```python
from build123d import *

# Parameters (mm, degrees)
P_IDAT_VYSUNUT_M1_DEPTH  = 22
ZAOBLIT1_R               = 3
SKICA2_W                 = 107.918638888
SKICA2_H                 = 41.380791124
P_IDAT_VYSUNUT_M2_DEPTH  = 2
SKICA3_R                 = 2.425
ODEBRAT_VYSUNUT_M1_DEPTH = 8.5


with BuildPart() as part:
    # Skica1 → Přidat vysunutím1 (new body)
    with BuildSketch(Plane.XY):
        Polygon((0, 0), (101.3, 0), (99.05, 33.2), (2.25, 33.2), align=None)
    extrude(amount=P_IDAT_VYSUNUT_M1_DEPTH)

    # Zaoblit1
    zaoblit1_edges = [part.edges().sort_by_distance(p)[0] for p in [
        (2.25, 33.2, 11),
        (99.05, 33.2, 11),
    ]]
    fillet(zaoblit1_edges, radius=ZAOBLIT1_R)

    # Skica2 → Přidat vysunutím2 (add)
    with BuildSketch(Plane(origin=(0, 0, 0), x_dir=(-1, 0, 0), z_dir=(0, 0, -1))):
        with Locations((-50.804022796, 17.445366235)):
            Rectangle(SKICA2_W, SKICA2_H)
    extrude(amount=P_IDAT_VYSUNUT_M2_DEPTH)

    # Skica3 → Odebrat vysunutím1 (cut)
    with BuildSketch(Plane.XY.offset(22)):
        with Locations((57.79, 9.455)):
            Circle(SKICA3_R)
        with Locations(Location((43.51, 9.455, 0), (0, 0, 180))):
            Circle(SKICA3_R)
        with Locations(Location((57.79, 23.735, 0), (0, 0, 180))):
            Circle(SKICA3_R)
        with Locations((43.51, 23.735)):
            Circle(SKICA3_R)
    extrude(amount=-ODEBRAT_VYSUNUT_M1_DEPTH, mode=Mode.SUBTRACT)


solid = part.part
```
Geometry: final body of the model. Coordinates: model frame, mm. A direction names the side the tool comes from. Coordinates: 2 decimals unless noted, no trailing zeros. Order: outer loops, then holes, each group sorted by start corner. A loop starts at its lowest first (then second) coordinate and runs counter-clockwise, first axis right, second up. Notation, with made-up numbers: M -20,22.5 L 33,22.5 A16 cw 33,31.5 Z; hole C 53.5,-3 d11. An arc over 180 degrees is marked long. Answer in a Markdown table with one row per item. Add a question column.
Q1. Contact query for flat-ended pins moving along their axis: P1, Ø4, axis at x = 42.5, y = 10, coming from the +Z side; P2, Ø5, axis at x = 89, z = 10.5, coming from the +Y side; P3, Ø2.5, axis at x = 58, y = 24, coming from the +Z side; P4, Ø10, axis at y = 28.5, z = 16, coming from the +X side. Output: stop coordinate, or through.
Q2. Section query C-C on z = 9. Return the cut outline in (x, y).
Q3. Section query B-B on x = 43.51. Return the cut outline in (y, z), and give its area (3 significant figures).
Q4. Section query D-D on x = 28.5. Return the cut outline in (y, z).
Q5. Line query: L1, parallel to Y at x = 43.51, z = 19.5; L2, parallel to Y at x = 57, z = 16.25; L3, parallel to Y at x = 92, z = 17. Output: solid intervals per line, ascending.
Q6. Reachability of faces 4 (the flat face through (1.045, 15.414, 10.846)), 5 (the flat face through (44, 9, 13.5)), 6 (the flat face through (51, 33.2, 11)) from +Z, -Z, +X, -X, +Y, -Y: full face, straight path, thin tool, end or side. Return the list, or none.
Q7. Section query A-A on z = 16. Return the cut outline in (x, y) (3 decimals), and give its area (3 significant figures).
Q8. Mould query, pull axis X, two halves, no side actions, for faces 1 (the cylindrical face through (41.27, 10.38, 17.81)), 2 (the flat face through (100.284, 14.989, 10.846)), 3 (the flat face through (50, 0, 11)). Classes: released by +X, released by -X, zero draft, split by the parting line, or undercut.
Completed:
| question | item | result |
|---|---|---|
| 1 | P1 | stops at z = 22 |
| 1 | P2 | stops at y = 33.2 |
| 1 | P3 | stops at z = 13.5 |
| 1 | P4 | stops at x = 99.71 |
| 2 | outline | M 0,0 L 101.3,0 L 99.24,30.4 A3 ccw 96.25,33.2 L 5.05,33.2 A3 ccw 2.06,30.4 Z |
| 3 | outline | M -3.25,-2 L 38.14,-2 L 38.14,0 L 33.2,0 L 33.2,22 L 26.16,22 L 26.16,13.5 L 21.31,13.5 L 21.31,22 L 11.88,22 L 11.88,13.5 L 7.03,13.5 L 7.03,22 L 0,22 L 0,0 L -3.25,0 Z |
| 3 | area | 731 mm2 |
| 4 | outline | M -3.25,-2 L 38.14,-2 L 38.14,0 L 33.2,0 L 33.2,22 L 0,22 L 0,0 L -3.25,0 Z |
| 5 | L1 | y = 0 to 7.03, 11.88 to 21.31, 26.16 to 33.2 |
| 5 | L2 | y = 0 to 7.16, 11.75 to 21.44, 26.03 to 33.2 |
| 5 | L3 | y = 0 to 33.2 |
| 6 | face 4 | +Z, -X, +Y |
| 6 | face 5 | +Z |
| 6 | face 6 | +Z, +X, -X, +Y |
| 7 | outline | M 0,0 L 101.3,0 L 99.24,30.403 A3 ccw 96.246,33.2 L 5.054,33.2 A3 ccw 2.06,30.403 Z; hole C 43.51,9.455 d4.85; hole C 43.51,23.735 d4.85; hole C 57.79,9.455 d4.85; hole C 57.79,23.735 d4.85 |
| 7 | area | 3,210 mm2 |
| 8 | face 1 | undercut |
| 8 | face 2 | released by +X |
| 8 | face 3 | zero draft |
